Geometry: final body of the model. Coordinates: model frame, mm. Face numbers are marked on the shaded views. A direction names the side the tool comes from. Give positions to 0.01 mm unless a question says otherwise; leave off trailing zeros. Write each loop counter-clockwise with the first axis right and the second up, starting at its lowest first coordinate (ties: lowest second). Pieces come first, ordered by that corner, then holes. Notation, with made-up numbers: M 63,30 L 69,30 A23 cw 69,59 Z; hole C 70,12.25 d7. An arc over 180 degrees is marked long. Use one line per item in the form item = value. Start each with the question number.
Item 1: Access query for the marked faces 4, 5 and 6. Directions: +Z, -Z, +X, -X, +Y, -Y. A direction counts if a zero-diameter tool reaches every point of the face in a straight line with its end or side. Return the directions, or none.
Item 2: Section query B-B on z = 0. Return loops of the section in (x, y) (1 decimal), then the cut area to 3 significant figures.
Item 3: Material intervals for line 1 along X through (y, z) = (2.5, 1.75) (3 decimals); line 2 along X through (y, z) = (-0.5, 1); line 3 along Z through (x, y) = (9.5, -0.5), sorted ascending. Write a range as from..to.
Item 4: Section query C-C on z = 2.5. Return loops of the section in (x, y) (3 decimals).
Item 5: Pull-direction query (Y, two-part tool) for the marked faces 1, 2 and 3; classes: released by +Y, released by -Y, zero draft, split by the parting line, or undercut.
Item 6: Section query A-A on x = 21.5. Return loops of the section in (y, z) (1 decimal).
Item 7: Contact query for flat-ended pins moving along their axis: P1, Ø1.5, axis at y = 0.5, z = 0, coming from the -X side; P2, Ø3, axis at x = 24.5, y = 2.5, coming from the +Z side; P3, Ø1.5, axis at x = 17, y = -2, coming from the -Z side. Output: stop coordinate, or through.
Item 8: Section query D-D on z = -2.25. Return loops of the section in (x, y) (3 decimals).
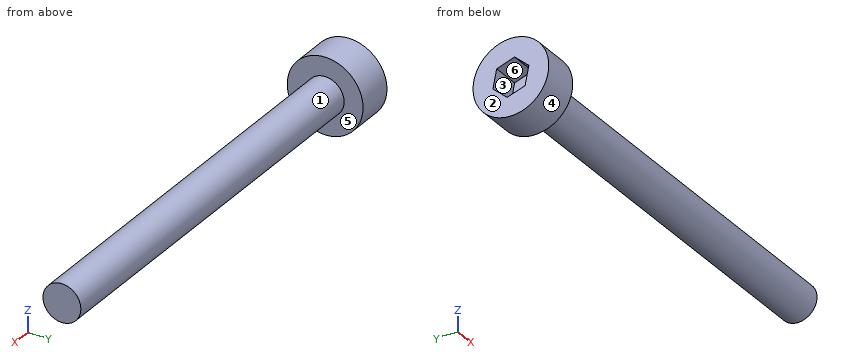
from build123d import *

# Parameters (mm, degrees)
F0_R     = 3.175
F1_DEPTH = 3.175
F2_R     = 1.5875
F3_DEPTH = 34.925
F4_DEPTH = 2.38125


with BuildPart() as f1:
    # F0 (on Right) → F1 (new body)
    with BuildSketch(Plane.YZ):
        Circle(F0_R)
        Polygon((1.193802, 1.046419), (1.503127, -0.510653), (0.309325, -1.557072), (-1.193802, -1.046419), (-1.503127, 0.510653), (-0.309325, 1.557072), align=None, mode=Mode.SUBTRACT)
        Polygon((0.309325, -1.557072), (1.503127, -0.510653), (1.193802, 1.046419), (-0.309325, 1.557072), (-1.503127, 0.510653), (-1.193802, -1.046419), align=None)
    extrude(amount=F1_DEPTH)

    # F2 (on face) → F3 (join)
    with BuildSketch(Plane.YZ.offset(3.175)):
        Circle(F2_R)
    extrude(amount=F3_DEPTH)

    # F0 (on Right) → F4 (cut)
    with BuildSketch(Plane.YZ):
        Polygon((0.309325, -1.557072), (1.503127, -0.510653), (1.193802, 1.046419), (-0.309325, 1.557072), (-1.503127, 0.510653), (-1.193802, -1.046419), align=None)
    extrude(amount=F4_DEPTH, mode=Mode.SUBTRACT)


solid = f1.part
Answer sheet:
q1.face_4 = +X, -X
q1.face_5 = +X
q1.face_6 = -X
q2.outline = M 0,-3.2 L 3.2,-3.2 L 3.2,-1.6 L 38.1,-1.6 L 38.1,1.6 L 3.2,1.6 L 3.2,3.2 L 0,3.2 L 0,1.4 L 2.4,1.4 L 2.4,-1.4 L 0,-1.4 Z
q2.area = 124 mm2
q3.line_1 = 0..3.175
q3.line_2 = 2.38..38.1
q3.line_3 = -1.51..1.51
q4.outline = M 0,-1.957 L 3.175,-1.957 L 3.175,1.957 L 0,1.957 Z
q5.face_1 = split by the parting line
q5.face_2 = zero draft
q5.face_3 = undercut
q6.outline = C 0,0 d3.2
q7.P1 = 2.38
q7.P2 = 1.23
q7.P3 = -0.98
q8.outline = M 0,-2.24 L 3.175,-2.24 L 3.175,2.24 L 0,2.24 Z
